Model file for the job. Use its own axes, mm. Face numbers are marked on the shaded views. A direction names the side the tool comes from. Round coordinates to 2 decimals unless told otherwise and drop trailing zeros. Loops run counter-clockwise (first coordinate to the right, second up) from the corner with the lowest first, then second, coordinate; pieces in that order, holes last. Notation, with made-up numbers: M 22,-16.5 L 64,-16.5 A32 cw 64,15.5 Z; hole C 58.25,-5 d1. An arc over 180 degrees is marked long. Use a Markdown table: item, result. Add a question column.
Q1. Probe line 1 (Z direction, x = 42.5, y = 1.5); line 2 (Z direction, x = 5, y = 2.75); line 3 (X direction, y = 10, z = -18.5). List the from-to ranges inside material, lowest first. Write a range as from..to.
Q2. Pin check, flat tips, straight feed: pin 1 (4 mm diameter, centred on y = 9.5, z = -9, fed in from -X); pin 2 (5 mm diameter, centred on x = -15, y = 5, fed in from -Z); pin 3 (8 mm diameter, centred on x = -38.5, y = 2.5, fed in from +Z); pin 4 (8 mm diameter, centred on x = -46.24, z = -33.59, fed in from -Y). Stop position of each tip, or through.
Q3. Mould opens along X. For the marked faces 1, 2, 3 and 4 say: +X half, -X half, draft (parallel to the pull), parting line (faces both ways), or undercut.
Q4. Cut at B-B (y = 12.5). Give the cut face in (x, z) (1 decimal).
Q5. Cut at A-A (z = 0). State how many separate pieces and enclosed holes the cut face has, plus the area to 3 significant figures.
Q6. Tool access for the marked faces 5 and 6: list every direction of +Z, -Z, +X, -X, +Y, -Y with a clear straight run to the whole face (end or side of a thin tool).
from build123d import *

# Parameters (mm, degrees)
SKETCH1_R                       = 61.9125
SKETCH1_R_2                     = 35.052
BOSS_EXTRUDE1_DEPTH             = 4.5212
SKETCH3_R                       = 52.3875
BOSS_EXTRUDE2_DEPTH             = 11.43
SKETCH4_R                       = 35.052
CUT_EXTRUDE1_DEPTH              = 89.998629731
SKETCH9_R                       = 36.000000009
CUT_EXTRUDE3_DEPTH              = 8.89
F_5_0MM_DOWEL_HOLE1_D           = 5
F_5_0MM_DOWEL_HOLE1_CSINK_D     = 5.05
F_5_0MM_DOWEL_HOLE1_CSINK_ANGLE = 90
CIRPATTERN1_COUNT               = 60
CUT_EXTRUDE5_DEPTH              = 89.998629731


with BuildPart() as part:
    # Sketch1 → Boss-Extrude1 (new body)
    with BuildSketch(Plane(origin=(0, 0, 0), x_dir=(1, 0, 0), z_dir=(0, 1, 0))):
        with Locations(Location((0, 0, 0), (0, 0, 270))):
            Circle(SKETCH1_R)
        with Locations(Location((0, -12.7, 0), (0, 0, 270))):
            Circle(SKETCH1_R_2, mode=Mode.SUBTRACT)
    extrude(amount=BOSS_EXTRUDE1_DEPTH)

    # Sketch3 → Boss-Extrude2 (add)
    with BuildSketch(Plane(origin=(0, 4.5212, 0), x_dir=(1, 0, 0), z_dir=(0, 1, 0))):
        with Locations(Location((0, 0, 0), (0, 0, 270))):
            Circle(SKETCH3_R)
    extrude(amount=BOSS_EXTRUDE2_DEPTH)

    # Sketch4 → Cut-Extrude1 (cut, through all)
    with BuildSketch(Plane.XZ):
        with Locations(Location((0, 12.7, 0), (0, 0, 270))):
            Circle(SKETCH4_R)
    extrude(amount=-CUT_EXTRUDE1_DEPTH, mode=Mode.SUBTRACT)

    # Sketch9 → Cut-Extrude3 (cut)
    with BuildSketch(Plane(origin=(0, 15.9512, 0), x_dir=(1, 0, 0), z_dir=(0, 1, 0))):
        with Locations(Location((0, -12.7, 0), (0, 0, 270))):
            Circle(SKETCH9_R)
    extrude(amount=-CUT_EXTRUDE3_DEPTH, mode=Mode.SUBTRACT)

    # Ø5.0mm Dowel Hole1 (through all)
    with Locations(Plane(origin=(0, 4.5212, 0), x_dir=(1, 0, 0), z_dir=(0, 1, 0))):
        with Locations((0, 57.15)):
            f_5_0mm_dowel_hole1 = CounterSinkHole(F_5_0MM_DOWEL_HOLE1_D / 2, F_5_0MM_DOWEL_HOLE1_CSINK_D / 2, counter_sink_angle=F_5_0MM_DOWEL_HOLE1_CSINK_ANGLE)

    # CirPattern1: Ø5.0mm Dowel Hole1 ×60 about axis
    cirpattern1_axis = Axis((0, 0, 0), (0, 1, 0))
    for i in range(1, CIRPATTERN1_COUNT):
        add(f_5_0mm_dowel_hole1.rotate(cirpattern1_axis, i * 360 / CIRPATTERN1_COUNT), mode=Mode.SUBTRACT)

    # Sketch10 → Cut-Extrude5 (cut, through all)
    with BuildSketch(Plane(origin=(0, 15.9512, 0), x_dir=(1, 0, 0), z_dir=(0, 1, 0))):
        with BuildLine():
            ThreePointArc((-27.568698422, 16.370448294), (0, 27.364000009), (27.568698422, 16.370448294))
            ThreePointArc((27.568698422, 16.370448294), (38.57955057, 16.056999754), (40.099152196, 26.966991775))
            ThreePointArc((40.099152196, 26.966991775), (0, 48.3235), (-40.099152196, 26.966991775))
            ThreePointArc((-40.099152196, 26.966991775), (-38.57955057, 16.056999754), (-27.568698422, 16.370448294))
        make_face()
    extrude(amount=-CUT_EXTRUDE5_DEPTH, mode=Mode.SUBTRACT)


solid = part.part
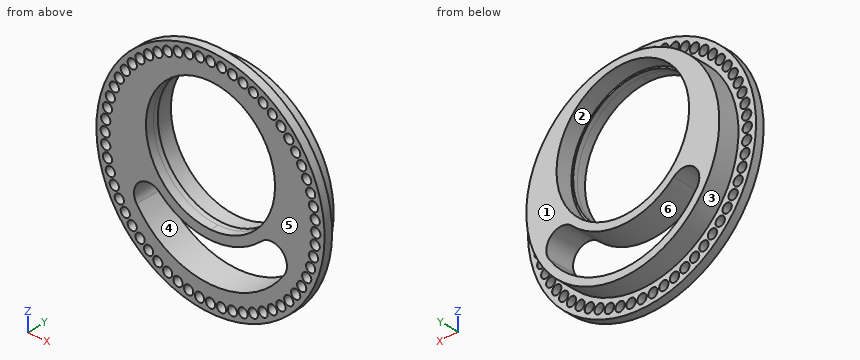
Checked values:
| question | item | result |
|---|---|---|
| 1 | line 1 | z = -45.02..-40.74, -35.74..35.74, 40.74..45.02 |
| 1 | line 2 | z = -61.71..-59.14, -54.53..-48.06, -27.05..-21.99, 47.39..54.53, 59.14..61.71 |
| 1 | line 3 | x = -49.01..-40.55, -25.13..-17.96, 17.96..25.13, 40.55..49.01 |
| 2 | pin 1 | stops at x = -51.92 |
| 2 | pin 2 | stops at z = -60.63 |
| 2 | pin 3 | stops at z = 51.41 |
| 2 | pin 4 | stops at y = 0 |
| 3 | face 1 | draft |
| 3 | face 2 | undercut |
| 3 | face 3 | parting line |
| 3 | face 4 | undercut |
| 4 | outline | C 0,0 d104.8; hole M -40.1,-27 A48.3 ccw 40.1,-27 A8.3 ccw 27.6,-16.4 A40.1 cw -27.6,-16.4 A8.3 ccw Z; hole C 0,12.7 d72 |
| 5 | separate pieces | 4 |
| 5 | enclosed holes | 0 |
| 5 | area | 652 mm^2 |
| 6 | face 5 | +Z, -Z, +X, -X, -Y |
| 6 | face 6 | +Y, -Y |
